Could you check a few things on this model? Use its own coordinates, in mm. Face numbers are marked on the shaded views. A direction names the side the tool comes from. Round coordinates to 2 decimals unless told otherwise and drop trailing zeros. Write each loop counter-clockwise with the first axis right and the second up, starting at its lowest first coordinate (ties: lowest second). Pieces come first, ordered by that corner, then holes.
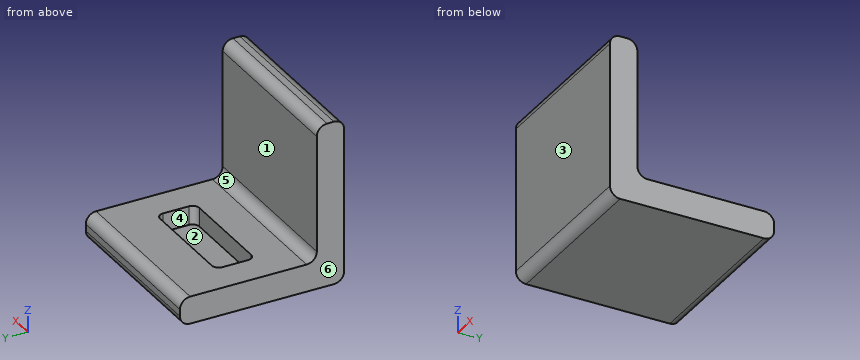
```python
from build123d import *

# Parameters (mm, degrees)
SKETCH1_W           = 50
SKETCH1_H           = 40
BOSS_EXTRUDE1_DEPTH = 8
SKETCH2_W           = 50
SKETCH2_H           = 48
BOSS_EXTRUDE2_DEPTH = 8
SKETCH3_W           = 31.5
SKETCH3_H           = 11.5
CUT_EXTRUDE1_DEPTH  = 5.5
FILLET1_R           = 2
FILLET2_R           = 3


with BuildPart() as part:
    # Sketch1 → Boss-Extrude1 (new body)
    with BuildSketch(Plane(origin=(0, 0, 0), x_dir=(1, 0, 0), z_dir=(0, 1, 0))):
        with Locations((0, 20)):
            Rectangle(SKETCH1_W, SKETCH1_H)
    extrude(amount=BOSS_EXTRUDE1_DEPTH)

    # Sketch2 → Boss-Extrude2 (add)
    with BuildSketch(Plane(origin=(0, 0, -40), x_dir=(-1, 0, 0), z_dir=(0, 0, -1))):
        with Locations((0, 24)):
            Rectangle(SKETCH2_W, SKETCH2_H)
    extrude(amount=BOSS_EXTRUDE2_DEPTH)

    # Sketch3 → Cut-Extrude1 (cut)
    with BuildSketch(Plane.XY.offset(-40)):
        with Locations((0, 26.75)):
            Rectangle(SKETCH3_W, SKETCH3_H)
    extrude(amount=-CUT_EXTRUDE1_DEPTH, mode=Mode.SUBTRACT)

    # Fillet1
    fillet1_edges = [part.edges().sort_by_distance(p)[0] for p in [
        (-15.75, 21, -42.75),
        (-15.75, 32.5, -42.75),
        (15.75, 32.5, -42.75),
        (15.75, 21, -42.75),
    ]]
    fillet(fillet1_edges, radius=FILLET1_R)

    # Fillet2
    fillet2_edges = [part.edges().sort_by_distance(p)[0] for p in [
        (0, 48, -40),
        (0, 0, -48),
        (0, 8, -40),
        (0, 48, -48),
        (0, 0, 0),
        (0, 8, 0),
    ]]
    fillet(fillet2_edges, radius=FILLET2_R)


solid = part.part
```
Q1. Imagine slicing it at D-D, the plane z = -10.5. Write out the boundary of the cut face in (x, y), then the cut area to 3 significant figures.
Q2. Imagine slicing it at A-A, the plane z = -44. Write out the boundary of the cut face in (x, y).
Q3. If I drill on L1, parallel to X at y = 29, z = -43; L2, parallel to Z at x = 21, y = 29; L3, parallel to Y at x = -10.5, z = -5, over which ranges is the centre line in solid material (lowest first)?
Q4. On a 3-axis mill with a long thin cutter (end or side, diameter ignored), from which of +Z, -Z, +X, -X, +Y, -Y can I reach the whole of each face in a straight line? I mean the marked faces 1, 2 and 3. Say none if no direction works.
Q5. I'm going to push flat-ended pins straight in: pin 1 Ø4 at (x, z) = (18, -34.5) entering from +Y; pin 2 Ø8 at (x, z) = (19, -34.5) entering from +Y; pin 3 Ø12.5 at (x, y) = (4, 29.5) entering from +Z. Where does each tip first touch, or does it pass through?
Q6. Imagine slicing it at C-C, the plane y = 19. Write out the boundary of the cut face in (x, z).
Q7. Imagine slicing it at B-B, the plane x = 0. Write out the boundary of the cut face in (y, z), then the cut area to 3 significant figures.
Q8. We'd pull the mould along X, two halves only. Please class the marked faces 4, 5 and 6: pulls with the +X half, pulls with the -X half, needs draft (parallel to the pull), parting line crosses it, or undercut.
Results found:
1. outline: (-25, 0) - (25, 0) - (25, 8) - (-25, 8) - close
1. area: 400 mm2
2. outline: (-25, 0) - (25, 0) - (25, 48) - (-25, 48) - close; hole (-15.75, 23) arc R2 ccw to (-13.75, 21) - (13.75, 21) arc R2 ccw to (15.75, 23) - (15.75, 30.5) arc R2 ccw to (13.75, 32.5) - (-13.75, 32.5) arc R2 ccw to (-15.75, 30.5) - close
3. L1: x = -25 to -15.75, 15.75 to 25
3. L2: z = -48 to -40
3. L3: y = 0 to 8
4. face 1: +Z, +X, -X, +Y
4. face 2: +Z
4. face 3: +Z, -Z, +X, -X, -Y
5. pin 1: stops at y = 8
5. pin 2: stops at y = 8.4
5. pin 3: stops at z = -40
6. outline: (-25, -48) - (25, -48) - (25, -40) - (-25, -40) - close
7. outline: (0, -45) arc R3 ccw to (3, -48) - (45, -48) arc R3 ccw to (48, -45) - (48, -43) arc R3 ccw to (45, -40) - (32.5, -40) - (32.5, -45.5) - (21, -45.5) - (21, -40) - (11, -40) arc R3 cw to (8, -37) - (8, -3) arc R3 ccw to (5, 0) - (3, 0) arc R3 ccw to (0, -3) - close
7. area: 633 mm2
8. face 4: undercut
8. face 5: needs draft
8. face 6: pulls with the -X half
